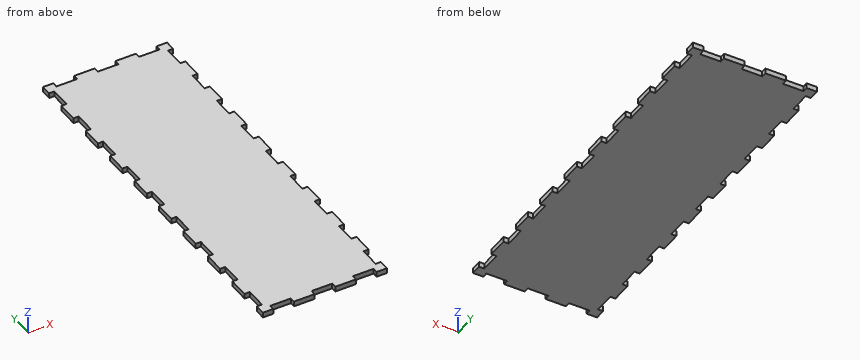
from build123d import *

# Parameters (mm, degrees)
SKETCH1_W            = 76.2
SKETCH1_H            = 228.6
EXTRUDE1_DEPTH       = 3.175
SKETCH3_W            = 3.175
SKETCH3_H            = 12.7
CUT_EXTRUDE1_DEPTH   = 3.175
LPATTERN1_COUNT      = 9
LPATTERN1_PITCH      = 25.4
LPATTERN1_COUNT_DIR2 = 2
LPATTERN1_PITCH_DIR2 = 73.025
SKETCH4_W            = 12.7
SKETCH4_H            = 3.175
CUT_EXTRUDE2_DEPTH   = 3.175
LPATTERN2_COUNT      = 3
LPATTERN2_PITCH      = 25.4
LPATTERN2_COUNT_DIR2 = 2
LPATTERN2_PITCH_DIR2 = 225.425


with BuildPart() as part:
    # Sketch1 → Extrude1 (new body)
    with BuildSketch(Plane.XY):
        with Locations((38.1, 114.3)):
            Rectangle(SKETCH1_W, SKETCH1_H)
    extrude(amount=EXTRUDE1_DEPTH)

    # Sketch3 → Cut-Extrude1 (cut)
    with BuildSketch(Plane.XY.offset(3.175)):
        with Locations((74.6125, 215.9)):
            Rectangle(SKETCH3_W, SKETCH3_H)
    cut_extrude1 = extrude(amount=-CUT_EXTRUDE1_DEPTH, mode=Mode.SUBTRACT)

    # LPattern1: Cut-Extrude1 9 × 2
    with Locations(*[(-j * LPATTERN1_PITCH_DIR2, -i * LPATTERN1_PITCH, 0) for i in range(LPATTERN1_COUNT) for j in range(LPATTERN1_COUNT_DIR2) if (i, j) != (0, 0)]):
        add(cut_extrude1, mode=Mode.SUBTRACT)

    # Sketch4 → Cut-Extrude2 (cut)
    with BuildSketch(Plane.XY.offset(3.175)):
        with Locations((63.5, 227.0125)):
            Rectangle(SKETCH4_W, SKETCH4_H)
    cut_extrude2 = extrude(amount=-CUT_EXTRUDE2_DEPTH, mode=Mode.SUBTRACT)

    # LPattern2: Cut-Extrude2 3 × 2
    with Locations(*[(-i * LPATTERN2_PITCH, -j * LPATTERN2_PITCH_DIR2, 0) for i in range(LPATTERN2_COUNT) for j in range(LPATTERN2_COUNT_DIR2) if (i, j) != (0, 0)]):
        add(cut_extrude2, mode=Mode.SUBTRACT)


solid = part.part
Source: CAD feature listing. Evaluate the final solid. Frame: model axes, mm. Give positions to 0.01 mm unless a question says otherwise; leave off trailing zeros. Write each loop counter-clockwise with the first axis right and the second up, starting at its lowest first coordinate (ties: lowest second). Pieces come first, ordered by that corner, then holes. Notation, with made-up numbers: M 62.25,42.25 L 79.25,42.25 A20 cw 79.25,73.25 Z; hole C 44,-33.75 d8. An arc over 180 degrees is marked long. Return JSON: item names as keys, results as strings. Group by question number.
1) Cut plane B-B, the plane x = 13. Output: boundary loops of the cut face in (y, z) (3 decimals), plus the area to 3 significant figures.
2) Cut plane A-A, the plane y = 62.5. Output: boundary loops of the cut face in (x, z) (3 decimals), plus the area to 3 significant figures.
3) Pin query (flat end, axial travel): P1, Ø1.6, axis at y = 138.5, z = 1, coming from the +X side (3 decimals); P2, Ø12, axis at x = 46, y = 24, coming from the -Z side; P3, Ø1, axis at x = 13.5, z = 1, coming from the -Y side (3 decimals). Return the tip coordinate at first contact, or that it passes through.
4) Material intervals for line 1 along X through (y, z) = (66, 0.9) (3 decimals); line 2 along Y through (x, z) = (65.5, 1.9) (3 decimals), sorted ascending. Write a range as [from, to].
Recorded:
{
 "1": {"outline": "M 3.175,0 L 225.425,0 L 225.425,3.175 L 3.175,3.175 Z", "area": "706 mm²"},
 "2": {"outline": "M 3.175,0 L 73.025,0 L 73.025,3.175 L 3.175,3.175 Z", "area": "222 mm²"},
 "3": {"P1": "stops at x = 73.025", "P2": "stops at z = 0", "P3": "stops at y = 3.175"},
 "4": {"line 1": "x = [3.175, 73.025]", "line 2": "y = [3.175, 225.425]"}
}
